```python
from build123d import *

# Parameters (mm, degrees)
SKETCH1_W           = 25.4
SKETCH1_H           = 203.2
BOSS_EXTRUDE1_DEPTH = 6.35
SKETCH2_R           = 5
CUT_EXTRUDE1_DEPTH  = 103.587389576
CUT_EXTRUDE2_DEPTH  = 103.587389576


with BuildPart() as part:
    # Sketch1 → Boss-Extrude1 (new body)
    with BuildSketch(Plane(origin=(0, 0, 0), x_dir=(1, 0, 0), z_dir=(0, 1, 0))):
        Rectangle(SKETCH1_W, SKETCH1_H)
    extrude(amount=BOSS_EXTRUDE1_DEPTH)

    # Sketch2 → Cut-Extrude1 (cut, through all)
    with BuildSketch(Plane(origin=(0, 6.35, 0), x_dir=(1, 0, 0), z_dir=(0, 1, 0))):
        with Locations(Location((0, -80, 0), (0, 0, 270))):
            Circle(SKETCH2_R)
        with Locations(Location((0, 80, 0), (0, 0, 270))):
            Circle(SKETCH2_R)
    extrude(amount=-CUT_EXTRUDE1_DEPTH, mode=Mode.SUBTRACT)

    # Sketch3 → Cut-Extrude2 (cut, through all)
    with BuildSketch(Plane(origin=(0, 6.35, 0), x_dir=(1, 0, 0), z_dir=(0, 1, 0))):
        with BuildLine():
            Line((6, 50.8), (6, -50.8))
            ThreePointArc((6, -50.8), (0, -56.8), (-6, -50.8))
            Line((-6, -50.8), (-6, 50.8))
            ThreePointArc((-6, 50.8), (0, 56.8), (6, 50.8))
        make_face()
    extrude(amount=-CUT_EXTRUDE2_DEPTH, mode=Mode.SUBTRACT)


solid = part.part
```
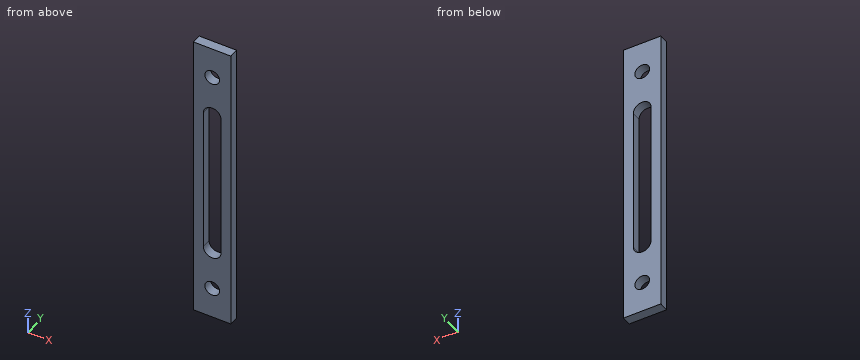
Check sheet for the modelled part. Datum: model origin and axes. Units: mm. Give positions to 0.01 mm unless a question says otherwise; leave off trailing zeros. Loops run counter-clockwise (first coordinate to the right, second up) from the corner with the lowest first, then second, coordinate; pieces in that order, holes last. Notation, with made-up numbers: M 68.25,44.5 L 73.25,44.5 A20 cw 73.25,48.5 Z; hole C -2,-32 d8. An arc over 180 degrees is marked long. Answer in a Markdown table with one row per item.
1) Cross-section at B-B (z = -17.5). Enter the section's corners in (x, y), plus the area to 3 significant figures.
Solutions:
| item | result |
|---|---|
| outline | M -12.7,0 L -6,0 L -6,6.35 L -12.7,6.35 Z; M 6,0 L 12.7,0 L 12.7,6.35 L 6,6.35 Z |
| area | 85.1 mm^2 |
2) Thickness scan on line 1 (X direction, y = 0.75, z = -43.5); line 2 (X direction, y = 2.75, z = -80); line 3 (Z direction, x = -0.75, y = 3). Record the ranges inside material, lowest first.
Solutions:
| item | result |
|---|---|
| line 1 | x = -12.7 to -6, 6 to 12.7 |
| line 2 | x = -12.7 to -5, 5 to 12.7 |
| line 3 | z = -101.6 to -84.94, -75.06 to -56.75, 56.75 to 75.06, 84.94 to 101.6 |
3) Cross-section at A-A (x = 0). Enter the section's corners in (y, z), plus the area to 3 significant figures.
Solutions:
| item | result |
|---|---|
| outline | M 0,-101.6 L 6.35,-101.6 L 6.35,-85 L 0,-85 Z; M 0,-75 L 6.35,-75 L 6.35,-56.8 L 0,-56.8 Z; M 0,56.8 L 6.35,56.8 L 6.35,75 L 0,75 Z; M 0,85 L 6.35,85 L 6.35,101.6 L 0,101.6 Z |
| area | 442 mm^2 |
4) Cross-section at C-C (y = 3.5). Enter the section's corners in (x, z), plus the area to 3 significant figures.
Solutions:
| item | result |
|---|---|
| outline | M -12.7,-101.6 L 12.7,-101.6 L 12.7,101.6 L -12.7,101.6 Z; hole M -6,-50.8 A6 ccw 6,-50.8 L 6,50.8 A6 ccw -6,50.8 Z; hole C 0,-80 d10; hole C 0,80 d10 |
| area | 3,670 mm^2 |
5) Cross-section at D-D (z = -80). Enter the section's corners in (x, y).
Solutions:
| item | result |
|---|---|
| outline | M -12.7,0 L -5,0 L -5,6.35 L -12.7,6.35 Z; M 5,0 L 12.7,0 L 12.7,6.35 L 5,6.35 Z |
